Design review of the part shown in the three views and the two pictorial views. Dimensions are in mm from the part's minimum x, y and z. Coordinates: 2 decimals unless noted, no trailing zeros. Order: outer loops, then holes, each group sorted by start corner. A loop starts at its lowest first (then second) coordinate and runs counter-clockwise, first axis right, second up. Notation, with made-up numbers: M 33,30.25 L 65,30.25 A21 cw 65,45.25 Z; hole C 82.5,22 d3. An arc over 180 degrees is marked long. Use CSV: the item, a comma, the result in double quotes.
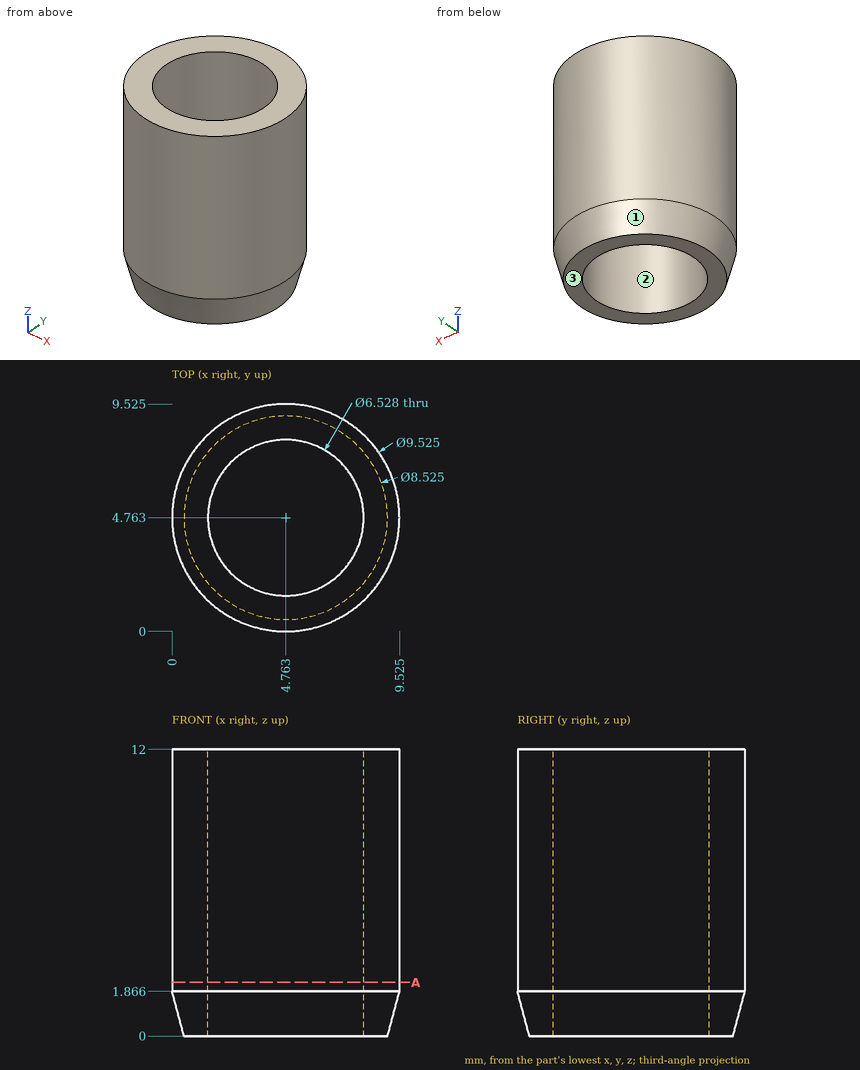
(1) Add section A-A on z = 2.25. State the section outline as (x, y) points (1 decimal).
The answers:
outline,"C 4.8,4.8 d9.5; hole C 4.8,4.8 d6.5"
(2) The part is to be moulded in two halves that separate along Y. For the marked faces 1, 2 and 3, say which applies: pulls with the +Y half, pulls with the -Y half, needs draft (parallel to the pull), parting line crosses it, or undercut.
The answers:
face 1,"parting line crosses it"
face 2,"undercut"
face 3,"needs draft"
(3) Clearance check with flat-ended pins moving along their axes: P1, Ø1, axis at x = 6, z = 8.5, coming from the +Y side; P2, Ø3, axis at x = 2.5, z = 3, coming from the -Y side; P3, Ø2, axis at y = 6.5, z = 4.5, coming from the +X side. State where each tip first meets the part, or that it passes through.
The answers:
P1,"stops at y = 9.47"
P2,"stops at y = 0.06"
P3,"stops at x = 9.47"
(4) Wall thickness on probe 1 along X at (y, z) = (4.75, 9.75) (1 decimal); probe 2 along X at (y, z) = (2, 5.25) (1 decimal): over which ranges is each line inside the solid? List them lowest first.
The answers:
probe 1,"x = 0 to 1.5, 8 to 9.5"
probe 2,"x = 0.9 to 3, 6.5 to 8.6"
